```python
from build123d import *

# Parameters (mm, degrees)
SKETCH1_R           = 1.5
SKETCH1_R_2         = 3.5
SKETCH1_R_3         = 1
SKETCH1_W           = 8
SKETCH1_H           = 4
BOSS_EXTRUDE1_DEPTH = 1


with BuildPart() as part:
    # Sketch1 → Boss-Extrude1 (new body)
    with BuildSketch(Plane.XY):
        with BuildLine():
            Line((-4.12667801, 12.25), (5.87332199, 12.25))
            Line((5.87332199, 12.25), (40.87332199, 12.25))
            Line((40.87332199, 12.25), (40.87332199, 10))
            ThreePointArc((40.87332199, 10), (50.867066736, -0.353646663), (40.166471095, -9.974986808))
            Line((40.166471095, -9.974986808), (40.166471095, -12.25))
            Line((40.166471095, -12.25), (5.87332199, -12.25))
            Line((5.87332199, -12.25), (-4.12667801, -12.25))
            Line((-4.12667801, -12.25), (-24.12667801, -12.25))
            Line((-24.12667801, -12.25), (-24.12667801, -8.25))
            Line((-24.12667801, -8.25), (2.87332199, -8.25))
            Line((2.87332199, -8.25), (2.87332199, 8.25))
            Line((2.87332199, 8.25), (-24.12667801, 8.25))
            Line((-24.12667801, 8.25), (-24.12667801, 12.25))
            Line((-24.12667801, 12.25), (-4.12667801, 12.25))
        make_face()
        with Locations((40.166439084, 6.964216866)):
            Circle(SKETCH1_R, mode=Mode.SUBTRACT)
        with Locations((47.837538856, 0.706882906)):
            Circle(SKETCH1_R, mode=Mode.SUBTRACT)
        with Locations((41.580204896, -6.964216866)):
            Circle(SKETCH1_R, mode=Mode.SUBTRACT)
        with Locations((33.909105124, -0.706882906)):
            Circle(SKETCH1_R, mode=Mode.SUBTRACT)
        with Locations((40.87332199, 0)):
            Circle(SKETCH1_R_2, mode=Mode.SUBTRACT)
        with Locations((-2.12667801, 10)):
            Circle(SKETCH1_R_3, mode=Mode.SUBTRACT)
        with Locations((-2.12667801, -10)):
            Circle(SKETCH1_R_3, mode=Mode.SUBTRACT)
        with Locations((-22.12667801, 10)):
            Circle(SKETCH1_R_3, mode=Mode.SUBTRACT)
        with Locations((-22.12667801, -10)):
            Circle(SKETCH1_R_3, mode=Mode.SUBTRACT)
        with Locations((20.166471095, 7)):
            Rectangle(SKETCH1_W, SKETCH1_H, mode=Mode.SUBTRACT)
        with Locations((20.166471095, -7)):
            Rectangle(SKETCH1_W, SKETCH1_H, mode=Mode.SUBTRACT)
    extrude(amount=BOSS_EXTRUDE1_DEPTH)


solid = part.part
```
Design review of the part built by this model. Coordinates are the model's own, in mm. Give positions to 0.01 mm unless a question says otherwise; leave off trailing zeros. Write each loop counter-clockwise with the first axis right and the second up, starting at its lowest first coordinate (ties: lowest second). Pieces come first, ordered by that corner, then holes. Notation, with made-up numbers: (76, 47.5) - (93, 47.5) arc R22 ccw to (93, 55.5) - close; hole circle Ø4 at (0, -9.75). An arc over 180 degrees is marked (long way). Return JSON: item names as keys, results as strings. Group by question number.
(1) Insertion check: pin 1 (1.8 mm diameter, centred on x = 47.84, y = 0.71, fed in from +Z); pin 2 (0.5 mm diameter, centred on y = -6.5, z = 0.5, fed in from +X). Each pin has a flat end and moves straight along its axis. Give the tip position at first contact, or say it passes through.
(2) We need section D-D, the plane z = 0.3. Give the number of separate pieces and of enclosed holes in the cut face, then the cut area to 3 significant figures.
(3) We need section C-C, the plane y = 0. Give the boundary of the cut face in (x, z), then the cut area to 3 significant figures.
(4) We need section B-B, the plane x = -11. Give the boundary of the cut face in (y, z).
(5) Mouldability with a two-part tool opening along Y and no side actions: class faces 1 (the flat face through (22, 0, 0)), 2 (the cylindrical face through (41.552, 6.39, 0.493)), 3 (the cylindrical face through (50.872, -0.129, 0.493)) as +Y half, -Y half, draft (parallel to the pull), parting line (faces both ways), or undercut.
(6) To check wall thickness, follow probe 1 along Y at (x, z) = (22, 0.2); probe 2 along Y at (x, z) = (-8.5, 0.5); probe 3 along X at (y, z) = (-6.5, 0.8). State the ranges of each line that lie inside material, in increasing order.
(7) We need section A-A, the plane x = 19.5. Give the boundary of the cut face in (y, z), then the cut area to 3 significant figures.
Reported:
{
 "1": {"pin 1": "passes through", "pin 2": "stops at x = 48.68"},
 "2": {"separate pieces": "1", "enclosed holes": "11", "area": "1,160 mm2"},
 "3": {"outline": "(2.87, 0) - (32.59, 0) - (32.59, 1) - (2.87, 1) - close; (35.23, 0) - (37.37, 0) - (37.37, 1) - (35.23, 1) - close; (44.37, 0) - (46.51, 0) - (46.51, 1) - (44.37, 1) - close; (49.16, 0) - (50.87, 0) - (50.87, 1) - (49.16, 1) - close", "area": "35.7 mm2"},
 "4": {"outline": "(-12.25, 0) - (-8.25, 0) - (-8.25, 1) - (-12.25, 1) - close; (8.25, 0) - (12.25, 0) - (12.25, 1) - (8.25, 1) - close"},
 "5": {"face 1": "draft", "face 2": "undercut", "face 3": "parting line"},
 "6": {"probe 1": "y = -12.25 to -9, -5 to 5, 9 to 12.25", "probe 2": "y = -12.25 to -8.25, 8.25 to 12.25", "probe 3": "x = 2.87 to 16.17, 24.17 to 40.15, 43.01 to 48.47"},
 "7": {"outline": "(-12.25, 0) - (-9, 0) - (-9, 1) - (-12.25, 1) - close; (-5, 0) - (5, 0) - (5, 1) - (-5, 1) - close; (9, 0) - (12.25, 0) - (12.25, 1) - (9, 1) - close", "area": "16.5 mm2"}
}
